Source: CAD feature listing. Evaluate the final solid. Frame: model axes, mm. Give positions to 0.01 mm unless a question says otherwise; leave off trailing zeros. Write each loop counter-clockwise with the first axis right and the second up, starting at its lowest first coordinate (ties: lowest second). Pieces come first, ordered by that corner, then holes.
Autodesk Inventor part; units mm, degrees
ref_plane "YZ Plane" through (0, 0, 0) normal (1, 0, 0) x (0, 1, 0)
ref_plane "XZ Plane" through (0, 0, 0) normal (0, 1, 0) x (-1, 0, 0)
ref_plane "XY Plane" through (0, 0, 0) normal (0, 0, 1) x (1, 0, 0)
sketch "Sketch1" plane through (0, 0, 0) normal (0, 0, 1) x (1, 0, 0)
  line L0 (-9.019, 23.22) -> (15.981, 23.22)
  line L1 (15.981, 23.22) -> (15.981, -21.78)
  line L2 (15.981, -21.78) -> (-9.019, -21.78)
  line L3 (-9.019, -21.78) -> (-9.019, 23.22)
  line L4 (-5.6447, 21.5683) -> (14.3553, 21.5683)
  line L5 (14.3553, 21.5683) -> (14.3553, -20.4317)
  line L6 (14.3553, -20.4317) -> (-5.6447, -20.4317)
  line L7 (-5.6447, -20.4317) -> (-5.6447, 21.5683)
  line L8 (17.9795, 15.2281) -> (17.9795, -13.9821)
  line L9 (17.9795, 15.2281) -> (15.9795, 15.2281)
  line L10 (15.9795, 15.2281) -> (15.9795, 17.2281)
  line L11 (15.9795, 17.2281) -> (17.9795, 17.2281)
  line L12 (17.9795, 17.2281) -> (17.9795, 15.2281)
  line L13 (17.9795, -13.9821) -> (15.9795, -13.9821)
  line L14 (15.9795, -13.9821) -> (15.9795, -15.9821)
  line L15 (15.9795, -15.9821) -> (17.9795, -15.9821)
  line L16 (17.9795, -15.9821) -> (17.9795, -13.9821)
  point P0 (0, 0)
  dimension "d0" = 25
  dimension "d2" = 20
  dimension "d4" = 29.2102
  dimension "d5" = 2
  dimension "d6" = 2
  dimension "d7" = 2
  dimension "d8" = 2
extrude "Extrusion1" add sketch "Sketch1" along normal blind 2 contours L0 L1 L2 L3 | L11 L12 L9 L1 | L1 L13 L16 L15
sketch "Sketch2" plane through (0, 0, 2) normal (0, 0, 1) x (1, 0, 0)
  line L0 (-9.019, 23.22) -> (-9.019, -21.78)
  line L1 (-9.019, -21.78) -> (15.9746, -21.78)
  line L2 (15.9746, -21.78) -> (15.9746, -26.578)
  line L3 (15.9746, -26.578) -> (-9.019, -26.578)
  line L4 (-9.019, -26.578) -> (-9.019, -21.78)
  line L5 (-9.019, 23.22) -> (15.981, 23.22)
  line L6 (-9.019, 23.22) -> (15.9746, 23.22)
  line L7 (15.9746, 23.22) -> (15.9746, 27.9895)
  line L8 (15.9746, 27.9895) -> (-9.019, 27.9895)
  line L9 (-9.019, 27.9895) -> (-9.019, 23.22)
  point P0 (0, 0)
extrude "Extrusion2" add sketch "Sketch2" against normal blind 2
sketch "Sketch3" plane through (0, 0, 2) normal (0, 0, 1) x (1, 0, 0)
  line L0 (-5.6447, -20.4317) -> (14.3553, -20.4317)
  line L1 (14.3553, -20.4317) -> (14.3553, 21.5683)
  line L2 (-5.6447, -20.4317) -> (14.3553, -20.4317)
  line L3 (14.3553, -20.4317) -> (14.3553, -15.4317)
  line L4 (14.3553, -15.4317) -> (-5.6447, -15.4317)
  line L5 (-5.6447, -15.4317) -> (-5.6447, -20.4317)
  line L6 (-5.6447, 21.5683) -> (-5.6447, -20.4317)
  line L7 (-5.6447, 21.5683) -> (14.3553, 21.5683)
  line L8 (14.3553, 21.5683) -> (14.3553, 16.5683)
  line L9 (14.3553, 16.5683) -> (-5.6447, 16.5683)
  line L10 (-5.6447, 16.5683) -> (-5.6447, 21.5683)
  point P0 (0, 0)
  dimension "d13" = 5
  dimension "d14" = 5
extrude "Extrusion3" add sketch "Sketch3" against normal blind 2 contours L5 L4 L1 L0 | L6 L7 L1 L9
sketch "Sketch4" plane through (0, 0, 2) normal (0, 0, 1) x (1, 0, 0)
  point P0 (0, 0)
sketch "Sketch5" plane through (0, 0, 2) normal (0, 0, 1) x (1, 0, 0)
  line L0 (-5.6447, -15.4317) -> (14.3572, -15.4317)
  line L1 (14.3572, -15.4317) -> (14.3572, -16.4317)
  line L2 (14.3572, -16.4317) -> (-5.6447, -16.4317)
  line L3 (-5.6447, -16.4317) -> (-5.6447, -15.4317)
  line L4 (-5.6447, -15.4317) -> (-5.6447, 16.5683)
  line L5 (-5.6447, 16.5683) -> (14.3572, 16.5683)
  line L6 (14.3572, 16.5683) -> (14.3572, 17.5683)
  line L7 (14.3572, 17.5683) -> (-5.6447, 17.5683)
  line L8 (-5.6447, 17.5683) -> (-5.6447, 16.5683)
  point P0 (0, 0)
  dimension "d17" = 1
  dimension "d18" = 1
extrude "Extrusion4" cut sketch "Sketch5" against normal blind 2
sketch "Sketch6" plane through (0, 0, 2) normal (0, 0, 1) x (1, 0, 0)
  point P0 (0, 0)
sketch "Sketch7" plane through (0, 0, 2) normal (0, 0, 1) x (1, 0, 0)
  line L0 (-4.5311, 20.3235) -> (-2.5311, 20.3235)
  line L1 (-2.5311, 20.3235) -> (-2.5311, 18.3235)
  line L2 (-2.5311, 18.3235) -> (-4.5311, 18.3235)
  line L3 (-4.5311, 18.3235) -> (-4.5311, 20.3235)
  line L4 (-2.5311, 19.3235) -> (7.8219, 19.3235)
  line L5 (7.8219, 20.3235) -> (9.8242, 20.3235)
  line L6 (9.8242, 20.3235) -> (9.8242, 18.3235)
  line L7 (9.8242, 18.3235) -> (7.8219, 18.3235)
  line L8 (7.8219, 18.3235) -> (7.8219, 20.3235)
  point P0 (0, 0)
  dimension "d21" = 2
  dimension "d22" = 2
  dimension "d23" = 10.353
extrude "Extrusion5" cut sketch "Sketch7" against normal blind 10
sketch "Sketch8" plane through (0, 0, 2) normal (0, 0, 1) x (1, 0, 0)
  line L0 (14.3572, -16.4317) -> (-5.6447, -16.4317)
  line L1 (-4.3843, -16.4317) -> (-4.3843, -17.2017)
  line L2 (-4.3843, -17.2017) -> (-2.3843, -17.2017)
  line L3 (-2.3843, -17.2017) -> (-2.3843, -19.2017)
  line L4 (-2.3843, -19.2017) -> (-4.3843, -19.2017)
  line L5 (-4.3843, -19.2017) -> (-4.3843, -17.2017)
  line L6 (-2.3843, -18.2017) -> (7.9687, -18.2017)
  line L7 (7.9687, -17.2017) -> (9.9687, -17.2017)
  line L8 (9.9687, -17.2017) -> (9.9687, -19.2017)
  line L9 (9.9687, -19.2017) -> (7.9687, -19.2017)
  line L10 (7.9687, -19.2017) -> (7.9687, -17.2017)
  point P0 (0, 0)
  dimension "d26" = 0.77
  dimension "d27" = 2
  dimension "d28" = 2
  dimension "d29" = 10.353
  dimension "d30" = 2
extrude "Extrusion6" cut sketch "Sketch8" against normal blind 10
sketch "Sketch9" plane through (0, 0, 2) normal (0, 0, 1) x (1, 0, 0)
  point P0 (0, 0)
properties part number "openslotforclamp"
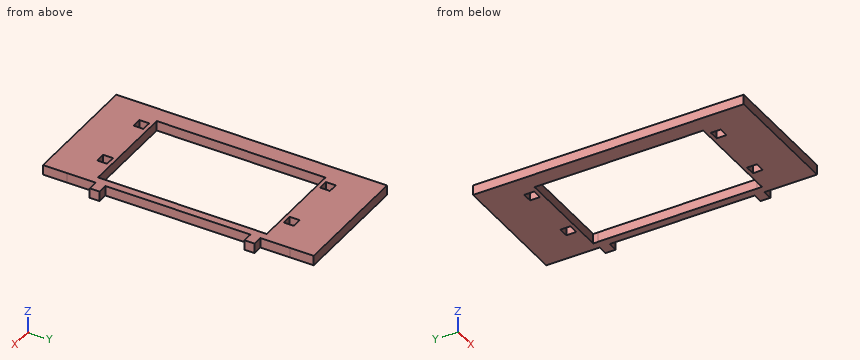
1. Pin query (flat end, axial travel): P1, Ø3, axis at x = 6.5, y = 14.5, coming from the +Z side; P2, Ø0.6, axis at y = -18, z = 0.5, coming from the +X side; P3, Ø1, axis at x = 17, z = 1.5, coming from the +Y side. Return the tip coordinate at first contact, or that it passes through.
2. Section query C-C (z = 0.8). Give the number of separate pieces and of enclosed holes in the cut face, plus the area to 3 significant figures.
3. Section query A-A (x = 10.75). Return loops of the section in (y, z), plus the area to 3 significant figures.
4. Section query D-D (y = -20.5). Return loops of the section in (x, z), plus the area to 3 significant figures.
5. Section query B-B (y = -11). Return loops of the section in (x, z).
6. Line query: probe 1 along Y at (x, z) = (8, 0.85); probe 2 along X at (y, z) = (-5, 1.7); probe 3 along Y at (x, z) = (2, 0.4). Output: solid intervals per line, ascending.
The answers:
1. P1: passes through
1. P2: stops at x = 15.98
1. P3: stops at y = 17.23
2. separate pieces: 1
2. enclosed holes: 5
2. area: 676 mm2
3. outline: (-26.58, 0) - (-16.43, 0) - (-16.43, 2) - (-26.58, 2) - close; (17.57, 0) - (27.99, 0) - (27.99, 2) - (17.57, 2) - close
3. area: 41.1 mm2
4. outline: (-9.02, 0) - (15.98, 0) - (15.98, 2) - (-9.02, 2) - close
4. area: 50.0 mm2
5. outline: (-9.02, 0) - (-5.64, 0) - (-5.64, 2) - (-9.02, 2) - close; (14.36, 0) - (15.98, 0) - (15.98, 2) - (14.36, 2) - close
6. probe 1: y = -26.58 to -19.2, -17.2 to -16.43, 17.57 to 18.32, 20.32 to 27.99
6. probe 2: x = -9.02 to -5.64, 14.36 to 15.98
6. probe 3: y = -26.58 to -16.43, 17.57 to 27.99
